CAD build for the part. Positions are in the model's coordinates, mm. Coordinates: 2 decimals unless noted, no trailing zeros. Loops run counter-clockwise (first coordinate to the right, second up) from the corner with the lowest first, then second, coordinate; pieces in that order, holes last. Notation, with made-up numbers: M 23,86 L 34,86 A29 ccw 34,113 Z; hole C 37,4.25 d11. An arc over 180 degrees is marked long. Answer as a JSON object with one key per item and string values. Group by question number.
Autodesk Inventor part; units mm, degrees
ref_plane "YZ Plane" through (0, 0, 0) normal (1, 0, 0) x (0, 1, 0)
ref_plane "XZ Plane" through (0, 0, 0) normal (0, 1, 0) x (-1, 0, 0)
ref_plane "XY Plane" through (0, 0, 0) normal (0, 0, 1) x (1, 0, 0)
sketch "Sketch1" plane through (0, 0, 0) normal (1, 0, 0) x (0, 1, 0)
  line L0 (0, 325) -> (0, 0)
  line L1 (0, 0) -> (-186, 0)
  line L2 (-186, 0) -> (-186, 85)
  line L3 (-2.414491, 325) -> (0, 325)
  line L4 (0, 325) -> (-95, 325)
  line L5 (-95, 325) -> (-186, 85)
  dimension "d0" = 325
  dimension "d1" = 186
  dimension "d2" = 85
  dimension "d3" = 95
  dimension "d33" = 240
  dimension "d34" = 91
extrude "Extrusion1" add sketch "Sketch1" along normal blind 6
sketch "Sketch2" plane through (6, 0, 0) normal (1, 0, 0) x (0, 0, -1)
  line L0 (-325, 0) -> (-325, -95)
  line L1 (-325, -8.1) -> (-331, -8.1)
  line L2 (-331, -8.1) -> (-331, -86.9)
  line L3 (-331, -86.9) -> (-325, -86.9)
  line L4 (-325, -86.9) -> (-325, -8.1)
  line L5 (-85, -186) -> (0, -186)
  line L6 (0, -186) -> (0, 0)
  line L7 (-76.9, -186) -> (-8.1, -186)
  line L8 (-8.1, -186) -> (-8.1, -192)
  line L9 (-8.1, -192) -> (-76.9, -192)
  line L10 (-76.9, -192) -> (-76.9, -186)
  line L11 (-325, -95) -> (-331, -86.9) construction
  line L12 (-325, 0) -> (-331, -8.1) construction
  dimension "d6" = 6
  dimension "d12" = 6
  dimension "d13" = 8.1
  dimension "d47" = 8.1
  dimension "d48" = 8.1
extrude "Extrusion2" add sketch "Sketch2" against normal blind 6
sketch "Sketch3" plane through (6, 0, 0) normal (1, 0, 0) x (0, 0, -1)
  line L0 (-317.426159, -97.871748) -> (-92.573841, -183.128252)
  line L1 (-92.573841, -183.128252) -> (-94.701061, -188.738504)
  line L2 (-94.701061, -188.738504) -> (-319.55338, -103.482)
  line L3 (-319.55338, -103.482) -> (-317.426159, -97.871748)
  line L4 (-325, -95) -> (-85, -186)
  dimension "d17" = 8.1
  dimension "d35" = 6
  dimension "d36" = 8.1
extrude "Extrusion3" add sketch "Sketch3" against normal blind 6
sketch "Sketch6" plane through (6, 0, 0) normal (1, 0, 0) x (0, 0, -1)
  line L0 (0, 0) -> (-325, 0)
  line L1 (0, -186) -> (0, 0)
  line L2 (0, -186) -> (-50, 25)
  line L3 (-50, 25) -> (0, 25)
  line L4 (0, 25) -> (0, -186)
  dimension "d38" = 50
  dimension "d39" = 25
extrude "Extrusion6" cut sketch "Sketch6" against normal through all
fillet "Fillet2" radius 3 4 edges at (3, 0, 325) (3, -95, 325) (3, -186, 85) (3, -186, 0)
fillet "Fillet3" radius 2 6 edges at (3, -192, 8.1) (3, -192, 76.9) (3, -188.7385, 94.7011) (3, -103.482, 319.5534) (3, -86.9, 331) (3, -8.1, 331)
sketch "Sketch4" plane through (6, 0, 0) normal (1, 0, 0) x (0, 0, -1)
  line L0 (-323.06361, -95.734214) -> (-85.513953, -185.805126)
  line L1 (-323.06361, -95.734214) -> (-85.513953, -185.805126)
  line L2 (-44.075829, 0) -> (-322, 0)
  line L3 (-325, -3) -> (-325, -8.1)
  line L4 (-325, -8.1) -> (-329, -8.1)
  line L5 (-305, -20) -> (-305, -81.193921)
  line L6 (-305, -81.193921) -> (-84.450343, -164.819)
  line L7 (-84.450343, -164.819) -> (-84.450343, -20)
  line L8 (-84.450343, -20) -> (-305, -20)
  arc A0 (-85.513953, -185.805126) -> (-84.450343, -186) centre (-84.450343, -183) ccw
  line L9 (-8.1, -186) -> (-3.79398, -186)
  point P0 (-191.521346, -165.651434)
  point P1 (-106.085382, -201.605735)
  point P2 (-3, 0)
  point P3 (0, 0)
  dimension "d24" = 20
  dimension "d26" = 20
  dimension "d27" = 20
extrude "Extrusion4" cut sketch "Sketch4" against normal through all
sketch "Sketch7" plane through (6, 0, 0) normal (1, 0, 0) x (0, 0, -1)
  line L0 (-84.450343, -20) -> (-84.450343, -164.819)
  line L1 (-0.874821, -182.308256) -> (-44.075829, 0)
  line L2 (-84.450343, -164.819) -> (-84.450343, -20)
  line L3 (-84.450343, -20) -> (-50.133044, -164.819)
  line L4 (-50.133044, -164.819) -> (-84.450343, -164.819)
  point P0 (0, 0)
extrude "Extrusion7" cut sketch "Sketch7" against normal through all
sketch "Sketch8" plane through (6, 0, 0) normal (1, 0, 0) x (0, 0, -1)
  line L0 (-84.450343, -20) -> (-50.133044, -164.819)
  line L1 (-50.133044, -164.819) -> (-84.450343, -164.819)
  line L2 (-305, -20) -> (-84.450343, -20)
  line L3 (-50.133044, -164.819) -> (-84.450343, -20)
  line L4 (-84.450343, -20) -> (-94.450343, -20)
  line L5 (-50.133044, -164.819) -> (-60.133044, -164.819)
  line L6 (-94.450343, -20) -> (-60.133044, -164.819)
  point P0 (0, 0)
  dimension "d44" = 10
extrude "Extrusion8" add sketch "Sketch8" against normal blind 6
fillet "Fillet4" radius 2 5 edges at (3, -164.819, 84.4503) (3, -164.819, 60.133) (3, -20, 94.4503) (3, -20, 305) (3, -81.1939, 305)
equation "\"d26\" = d24"
equation "\"d27\" = d24"
properties part number "TopSidePanel-Left"
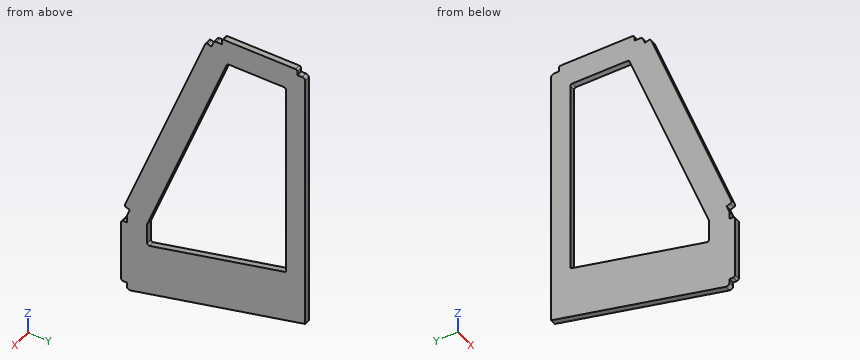
Item 1: Drill centre lines: L1, parallel to Z at x = 4.35, y = -42.5; L2, parallel to Y at x = 5.7, z = 259; L3, parallel to Z at x = 4, y = -21.5. Where is each one in solid material? Low to high. Write a range as from..to.
Item 2: Slice it at B-B, the plane y = -118. Write the cut outline in (x, z), then the cut area to 3 significant figures.
Item 3: Pin check, flat tips, straight feed: pin 1 (1.2 mm diameter, centred on x = 4.5, y = -189, fed in from -Z); pin 2 (1.8 mm diameter, centred on x = 3, z = 79, fed in from -Y); pin 3 (1.8 mm diameter, centred on x = 3, z = 78, fed in from +Y); pin 4 (3 mm diameter, centred on x = 3, z = 326, fed in from -Y). Stop position of each tip, or through.
Item 4: Slice it at A-A, the plane z = 71. Write the cut outline in (x, y).
Computed:
{
 "1": {"L1": "34..89.12, 305..331", "L2": "-126.44..-98.64, -20..0", "L3": "38.98..94.1, 304.94..331"},
 "2": {"outline": "M 0,16.11 L 6,16.11 L 6,71.23 L 0,71.23 Z; M 0,207.93 L 6,207.93 L 6,281.26 L 0,281.26 Z", "area": "771 mm2"},
 "3": {"pin 1": "z = 8.1", "pin 2": "y = -186", "pin 3": "y = 0", "pin 4": "y = -94.59"},
 "4": {"outline": "M 0,-192 L 6,-192 L 6,-164.82 L 0,-164.82 Z; M 0,-118.96 L 6,-118.96 L 6,0 L 0,0 Z"}
}
